Print and shaded views of the part. All mm, measured from the part's lowest x, y and z. Coordinates: 2 decimals unless noted, no trailing zeros. Write each loop counter-clockwise with the first axis right and the second up, starting at its lowest first coordinate (ties: lowest second). Pieces come first, ordered by that corner, then holes. Notation, with made-up numbers: (20, 4.25) -> (36, 4.25) arc R23 ccw to (36, 36.25) -> close; hole circle Ø1 at (33, 52). An arc over 180 degrees is marked (long way). Write item = value, one per line.
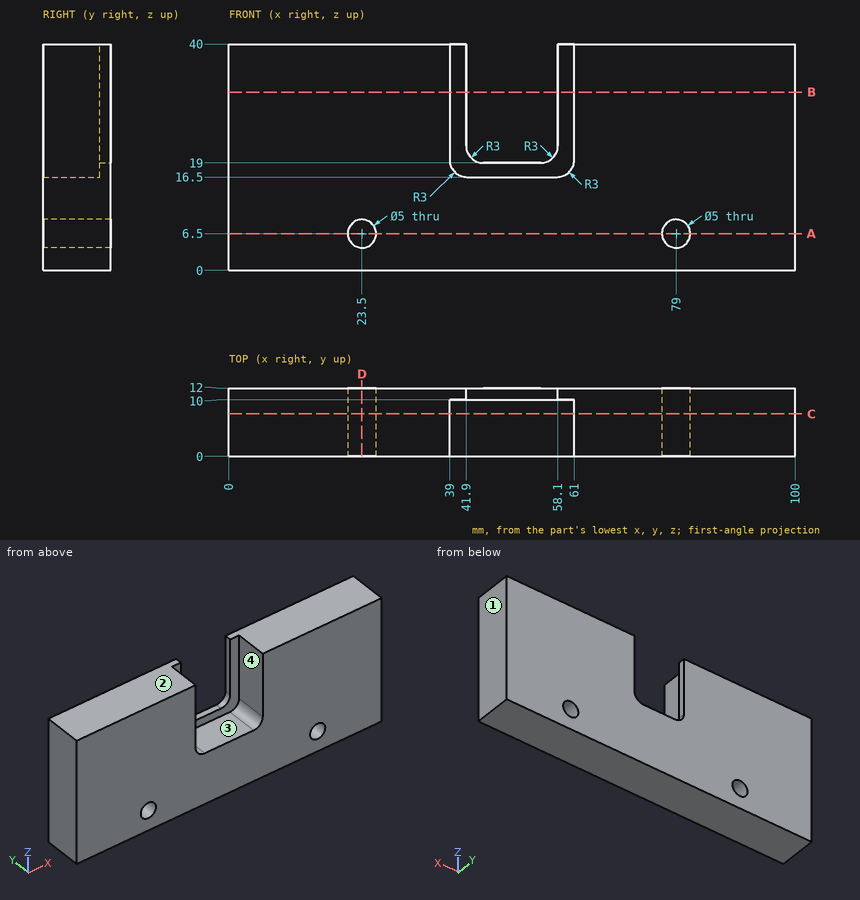
Q1. Pin check, flat tips, straight feed: pin 1 (5 mm diameter, centred on x = 44.5, z = 20.5, fed in from -Y); pin 2 (2 mm diameter, centred on x = 50, y = 10.5, fed in from +Z). Stop position of each tip, or through.
Model answer:
pin_1 = 10
pin_2 = 19
Q2. Probe line 1 (Z direction, x = 79, y = 9.25); line 2 (X direction, y = 6.5, z = 33.5); line 3 (Y direction, x = 40.5, z = 22.5). List the from-to ranges inside material, lowest first. Write a range as from..to.
Model answer:
line_1 = 0..4, 9..40
line_2 = 0..39, 61..100
line_3 = 10..12
Q3. Saw through at A-A on z = 6.5. Give the cut face in (x, y), and give its area (3 significant figures).
Model answer:
outline = (0, 0) -> (21, 0) -> (21, 12) -> (0, 12) -> close; (26, 0) -> (76.5, 0) -> (76.5, 12) -> (26, 12) -> close; (81.5, 0) -> (100, 0) -> (100, 12) -> (81.5, 12) -> close
area = 1,080 mm²
Q4. Saw through at D-D on x = 23.5. Give the cut face in (y, z), and give its area (3 significant figures).
Model answer:
outline = (0, 0) -> (12, 0) -> (12, 4) -> (0, 4) -> close; (0, 9) -> (12, 9) -> (12, 40) -> (0, 40) -> close
area = 420 mm²
Q5. Mould opens along X. For the marked faces 1, 2, 3 and 4 say: released by +X, released by -X, zero draft, split by the parting line, or undercut.
Model answer:
face_1 = released by +X
face_2 = zero draft
face_3 = undercut
face_4 = undercut
Q6. Saw through at B-B on z = 31.5. Give the cut face in (x, y), and give its area (3 significant figures).
Model answer:
outline = (0, 0) -> (39, 0) -> (39, 10) -> (41.9, 10) -> (41.9, 12) -> (0, 12) -> close; (58.1, 10) -> (61, 10) -> (61, 0) -> (100, 0) -> (100, 12) -> (58.1, 12) -> close
area = 948 mm²
Q7. Saw through at C-C on y = 7.5. Give the cut face in (x, z), and give its area (3 significant figures).
Model answer:
outline = (0, 0) -> (100, 0) -> (100, 40) -> (61, 40) -> (61, 19.5) arc R3 cw to (58, 16.5) -> (42, 16.5) arc R3 cw to (39, 19.5) -> (39, 40) -> (0, 40) -> close; hole circle Ø5 at (23.5, 6.5); hole circle Ø5 at (79, 6.5)
area = 3,450 mm²
